CAD build for the part. Positions are in the model's coordinates, mm. Coordinates: 2 decimals unless noted, no trailing zeros. Loops run counter-clockwise (first coordinate to the right, second up) from the corner with the lowest first, then second, coordinate; pieces in that order, holes last. Notation, with made-up numbers: (11, 15) -> (21, 15) arc R28 cw to (21, 54) -> close; hole circle Ø10 at (-5, -14.5). An arc over 180 degrees is marked (long way). Return JSON: item names as keys, results as strings. Group by question number.
(1) Saw through at B-B on x = 9. Give the number of separate pieces and of enclosed holes in the cut face, then the cut area to 3 significant figures.
(2) Saw through at A-A on z = 9. Write the cut outline in (x, y), then the cut area to 3 significant figures.
(3) Probe L1, parallel to Y at x = 4.5, z = 70.75; L2, parallel to Z at x = 6, y = 98.75; L3, parallel to X at y = 102, z = -46. List the from-to ranges inside material, lowest first.
(4) Saw through at C-C on y = -69.5. Write the cut outline in (x, z), then the cut area to 3 significant figures.
(5) Flat gauge pins, fed straight in: pin 1 Ø0.6 at (x, y) = (6.5, -41) entering from +Z; pin 2 Ø1 at (y, z) = (44.5, -5.5) entering from -X; pin 3 Ø3.5 at (x, z) = (7.5, -1) entering from +Y; pin 4 Ø1 at (x, z) = (7.5, -59) entering from -Y. Where does each tip first touch, or does it go through?
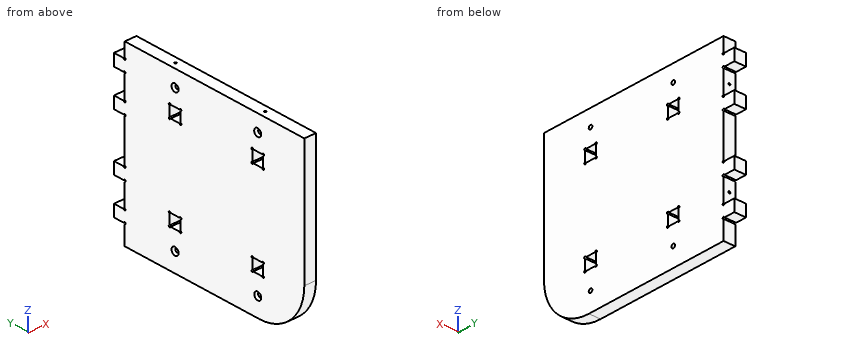
```python
from build123d import *

# Parameters (mm, degrees)
SKETCH1_R           = 2
SKETCH1_W           = 12.1
SKETCH1_H           = 12.1
BOSS_EXTRUDE1_DEPTH = 12
SKETCH2_R           = 0.9921875
CUT_EXTRUDE1_DEPTH  = 15
CUT_EXTRUDE2_START  = 108.950538
SKETCH4_R           = 0.9921875
CUT_EXTRUDE2_DEPTH  = 15
SKETCH5_R           = 1
CUT_EXTRUDE3_DEPTH  = 15


# Read off the part's stored shape, not the designer's step: AdvancedHole1
with BuildPart() as part:
    # Sketch1 → Boss-Extrude1 (new body)
    with BuildSketch(Plane(origin=(0, 0, 0), x_dir=(0, 0, -1), z_dir=(1, 0, 0))):
        with BuildLine():
            Line((-72.5, 120.950537961), (-72.5, 108.950537961))
            Line((-72.5, 108.950537961), (-87.5, 108.950537961))
            Line((-87.5, 108.950537961), (-87.5, -91.049462039))
            Line((-87.5, -91.049462039), (40.5, -91.049462039))
            ThreePointArc((40.5, -91.049462039), (75.855339059, -76.404801099), (90.5, -41.049462039))
            Line((90.5, -41.049462039), (90.5, 108.950537961))
            Line((90.5, 108.950537961), (70.5, 108.950537961))
            Line((70.5, 108.950537961), (70.5, 120.950537961))
            Line((70.5, 120.950537961), (58.5, 120.950537961))
            Line((58.5, 120.950537961), (58.5, 108.950537961))
            Line((58.5, 108.950537961), (33.5, 108.950537961))
            Line((33.5, 108.950537961), (33.5, 120.950537961))
            Line((33.5, 120.950537961), (21.5, 120.950537961))
            Line((21.5, 120.950537961), (21.5, 108.950537961))
            Line((21.5, 108.950537961), (-23.5, 108.950537961))
            Line((-23.5, 108.950537961), (-23.5, 120.950537961))
            Line((-23.5, 120.950537961), (-35.5, 120.950537961))
            Line((-35.5, 120.950537961), (-35.5, 108.950537961))
            Line((-35.5, 108.950537961), (-60.5, 108.950537961))
            Line((-60.5, 108.950537961), (-60.5, 120.950537961))
            Line((-60.5, 120.950537961), (-72.5, 120.950537961))
        make_face()
        with Locations((71.25, 52.900537961)):
            Circle(SKETCH1_R, mode=Mode.SUBTRACT)
        with Locations((71.25, -39.199462039)):
            Circle(SKETCH1_R, mode=Mode.SUBTRACT)
        with Locations((-70.75, 52.900537961)):
            Circle(SKETCH1_R, mode=Mode.SUBTRACT)
        with Locations((-70.75, -39.199462039)):
            Circle(SKETCH1_R, mode=Mode.SUBTRACT)
        with Locations((46, 52.900537961)):
            Rectangle(SKETCH1_W, SKETCH1_H, mode=Mode.SUBTRACT)
        with Locations((46, -39.199462039)):
            Rectangle(SKETCH1_W, SKETCH1_H, mode=Mode.SUBTRACT)
        with Locations((-48, 52.900537961)):
            Rectangle(SKETCH1_W, SKETCH1_H, mode=Mode.SUBTRACT)
        with Locations((-48, -39.199462039)):
            Rectangle(SKETCH1_W, SKETCH1_H, mode=Mode.SUBTRACT)
    extrude(amount=BOSS_EXTRUDE1_DEPTH)

    # Sketch2 → Cut-Extrude1 (cut)
    with BuildSketch(Plane.XY.offset(87.5)):
        with Locations((6, 58.950537961)):
            Circle(SKETCH2_R)
        with Locations((6, -41.049462039)):
            Circle(SKETCH2_R)
    extrude(amount=-CUT_EXTRUDE1_DEPTH, mode=Mode.SUBTRACT)

    # Sketch4 → Cut-Extrude2 (cut)
    with BuildSketch(Plane(origin=(0, 0, 0), x_dir=(1, 0, 0), z_dir=(0, 1, 0)).offset(CUT_EXTRUDE2_START)):
        with Locations(Location((6, 46, 0), (0, 0, 90))):
            Circle(SKETCH4_R)
        with Locations(Location((6, -48, 0), (0, 0, 90))):
            Circle(SKETCH4_R)
    extrude(amount=-CUT_EXTRUDE2_DEPTH, mode=Mode.SUBTRACT)

    # Sketch5 → Cut-Extrude3 (cut)
    with BuildSketch(Plane(origin=(0, 0, 0), x_dir=(0, 0, -1), z_dir=(1, 0, 0))):
        with Locations((-54.05, 58.950537961)):
            Circle(SKETCH5_R)
        with Locations((-41.95, 58.950537961)):
            Circle(SKETCH5_R)
        with Locations((-41.95, 46.850537961)):
            Circle(SKETCH5_R)
        with Locations((-54.05, 46.850537961)):
            Circle(SKETCH5_R)
        with Locations((39.95, 58.950537961)):
            Circle(SKETCH5_R)
        with Locations((52.05, 58.950537961)):
            Circle(SKETCH5_R)
        with Locations((52.05, 46.850537961)):
            Circle(SKETCH5_R)
        with Locations((39.95, 46.850537961)):
            Circle(SKETCH5_R)
        with Locations((-41.95, -33.149462039)):
            Circle(SKETCH5_R)
        with Locations((-54.05, -33.149462039)):
            Circle(SKETCH5_R)
        with Locations((-41.95, -45.249462039)):
            Circle(SKETCH5_R)
        with Locations((-54.05, -45.249462039)):
            Circle(SKETCH5_R)
        with Locations((39.95, -33.149462039)):
            Circle(SKETCH5_R)
        with Locations((52.05, -33.149462039)):
            Circle(SKETCH5_R)
        with Locations((52.05, -45.249462039)):
            Circle(SKETCH5_R)
        with Locations((39.95, -45.249462039)):
            Circle(SKETCH5_R)
        with Locations((21.5, 108.950537961)):
            Circle(SKETCH5_R)
        with Locations((33.5, 108.950537961)):
            Circle(SKETCH5_R)
        with Locations((58.5, 108.950537961)):
            Circle(SKETCH5_R)
        with Locations((70.5, 108.950537961)):
            Circle(SKETCH5_R)
        with Locations((-23.5, 108.950537961)):
            Circle(SKETCH5_R)
        with Locations((-35.5, 108.950537961)):
            Circle(SKETCH5_R)
        with Locations((-60.5, 108.950537961)):
            Circle(SKETCH5_R)
        with Locations((-72.5, 108.950537961)):
            Circle(SKETCH5_R)
    extrude(amount=CUT_EXTRUDE3_DEPTH, mode=Mode.SUBTRACT)

    # AdvancedHole1 outline → AdvancedHole1 (revolve, cut)
    with BuildSketch(Plane(origin=(0, -39.199462039, -71.25), x_dir=(0, 1, 0), z_dir=(0, 0, -1))):
        Polygon((3.8989, 0), (2, 2.184434568), (2, 0), align=None)
    revolve(axis=Axis((0, -39.199462039, -71.25), (1, 0, 0)), mode=Mode.SUBTRACT)

    # AdvancedHole1 2 outline → AdvancedHole1 2 (revolve, cut)
    with BuildSketch(Plane(origin=(0, -39.149462039, 70.75), x_dir=(0, 1, 0), z_dir=(0, 0, -1))):
        Polygon((3.8989, 0), (1.949985604, 2.24196955), (1.949985604, 0), align=None)
    revolve(axis=Axis((0, -39.149462039, 70.75), (1, 0, 0)), mode=Mode.SUBTRACT)

    # AdvancedHole1 3 outline → AdvancedHole1 3 (revolve, cut)
    with BuildSketch(Plane(origin=(0, 52.900537961, -71.25), x_dir=(0, 1, 0), z_dir=(0, 0, -1))):
        Polygon((3.8989, 0), (2, 2.184434568), (2, 0), align=None)
    revolve(axis=Axis((0, 52.900537961, -71.25), (1, 0, 0)), mode=Mode.SUBTRACT)

    # AdvancedHole1 4 outline → AdvancedHole1 4 (revolve, cut)
    with BuildSketch(Plane(origin=(0, 52.900537961, 70.75), x_dir=(0, 1, 0), z_dir=(0, 0, -1))):
        Polygon((3.8989, 0), (2, 2.184434568), (2, 0), align=None)
    revolve(axis=Axis((0, 52.900537961, 70.75), (1, 0, 0)), mode=Mode.SUBTRACT)


solid = part.part
```
Geometry results:
{
 "1": {"separate pieces": "1", "enclosed holes": "8", "area": "34,900 mm²"},
 "2": {"outline": "(0, -91.05) -> (12, -91.05) -> (12, 108.95) -> (0, 108.95) -> close", "area": "2,400 mm²"},
 "3": {"L1": "-91.05 to -41.2, -37.2 to 50.9, 54.9 to 120.95", "L2": "-90.5 to -46.99, -45.01 to 47.01, 48.99 to 87.5", "L3": "0 to 5.01, 6.99 to 12"},
 "4": {"outline": "(0, -81.62) -> (12, -81.62) -> (12, 87.5) -> (0, 87.5) -> close", "area": "2,030 mm²"},
 "5": {"pin 1": "z = 72.5", "pin 2": "x = 0", "pin 3": "y = 108.95", "pin 4": "y = -87.7"}
}
